```python
from build123d import *

# Parameters (mm, degrees)
SKETCH1_W           = 279.4
SKETCH1_H           = 165.1
BOSS_EXTRUDE1_DEPTH = 254
SKETCH2_R           = 38.8874
CUT_EXTRUDE1_DEPTH  = 413.114510786
SKETCH3_R           = 2.7686
CUT_EXTRUDE2_DEPTH  = 413.114510786


with BuildPart() as part:
    # Sketch1 → Boss-Extrude1 (new body)
    with BuildSketch(Plane.XY):
        with Locations((139.7, 82.55)):
            Rectangle(SKETCH1_W, SKETCH1_H)
    extrude(amount=BOSS_EXTRUDE1_DEPTH)

    # Sketch2 → Cut-Extrude1 (cut, through all)
    with BuildSketch(Plane.XY):
        with Locations((139.7, 0)):
            Circle(SKETCH2_R)
    extrude(amount=CUT_EXTRUDE1_DEPTH, mode=Mode.SUBTRACT)

    # Sketch3 → Cut-Extrude2 (cut, through all)
    with BuildSketch(Plane.XY):
        with Locations((6.35, 149.225)):
            Circle(SKETCH3_R)
        with Locations((139.7, 149.225)):
            Circle(SKETCH3_R)
        with Locations((273.05, 149.225)):
            Circle(SKETCH3_R)
        with Locations((6.35, 73.025)):
            Circle(SKETCH3_R)
        with Locations((273.05, 73.025)):
            Circle(SKETCH3_R)
        with Locations((6.35, 9.525)):
            Circle(SKETCH3_R)
        with Locations((273.05, 9.525)):
            Circle(SKETCH3_R)
    extrude(amount=CUT_EXTRUDE2_DEPTH, mode=Mode.SUBTRACT)


solid = part.part
```
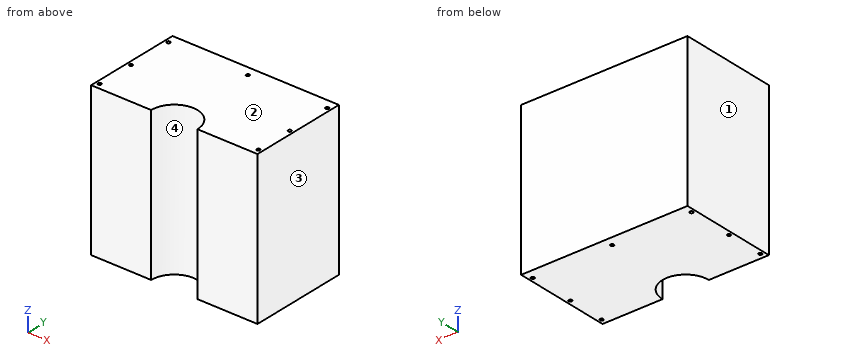
Can you work these out from the model? Positions are in its coordinate system, mm. Face numbers are marked on the shaded views. Give positions to 0.01 mm unless a question says otherwise; leave off trailing zeros. Loops run counter-clockwise (first coordinate to the right, second up) from the corner with the lowest first, then second, coordinate; pieces in that order, holes last. Notation, with made-up numbers: M 71.5,14.5 L 100.5,14.5 A22 ccw 100.5,21.5 Z; hole C 28.5,-21.5 d1. An arc over 180 degrees is marked long. Use one line per item in the form item = value. Start each with the question number.
(1) Thinking about a two-plate mould opening in X: for the marked faces 1, 2, 3 and 4, which applies, released by +X, released by -X, zero draft, split by the parting line, or undercut?
(2) I want a section at B-B, the plane z = 92. Write out the boundary of the cut face in (x, y) (3 decimals).
(3) I'm going to push a flat-ended pin straight in: P1, Ø3.5, axis at x = 6.35, y = 149.225, coming from the +Z side. Where does the tip first touch, or does it pass through?
(4) I want a section at C-C, the plane x = 147.5. Write out the boundary of the cut face in (y, z).
(5) I want a section at A-A, the plane y = 29. Write out the boundary of the cut face in (x, z), and give its area (3 significant figures).
(6) Please list where these lines run through material, in increasing order: line 1 (Y direction, x = 273.05, z = 190); line 2 (X direction, y = 73.5, z = 134); line 3 (X direction, y = 7.5, z = 241).
Worked out:
q1.face_1 = released by -X
q1.face_2 = zero draft
q1.face_3 = released by +X
q1.face_4 = undercut
q2.outline = M 0,0 L 100.813,0 A38.887 cw 178.587,0 L 279.4,0 L 279.4,165.1 L 0,165.1 Z; hole C 6.35,9.525 d5.537; hole C 6.35,73.025 d5.537; hole C 6.35,149.225 d5.537; hole C 139.7,149.225 d5.537; hole C 273.05,9.525 d5.537; hole C 273.05,73.025 d5.537; hole C 273.05,149.225 d5.537
q3.P1 = through
q4.outline = M 38.1,0 L 165.1,0 L 165.1,254 L 38.1,254 Z
q5.outline = M 0,0 L 113.79,0 L 113.79,254 L 0,254 Z; M 165.61,0 L 279.4,0 L 279.4,254 L 165.61,254 Z
q5.area = 57,800 mm²
q6.line_1 = 0 to 6.76, 12.29 to 70.26, 75.79 to 146.46, 151.99 to 165.1
q6.line_2 = 0 to 3.62, 9.08 to 270.32, 275.78 to 279.4
q6.line_3 = 0 to 4.46, 8.24 to 101.54, 177.86 to 271.16, 274.94 to 279.4
